```python
from build123d import *

# Parameters (mm, degrees)
SKETCH1_W                   = 14
SKETCH1_H                   = 16.3
SKETCH1_W_2                 = 10
SKETCH1_H_2                 = 13.3
SKETCH1_W_3                 = 9.5
SKETCH1_H_3                 = 7
CAP_EXTRUDE_DEPTH           = 1
SKETCH1_7_W                 = 14
SKETCH1_7_H                 = 5
FLAP_EXTRUDE_DEPTH          = 1.75
CUT_EXTRUDE2_REACH          = 3.75
SKETCH1_9_W                 = 9.5
SKETCH1_9_H                 = 7
F_1_5MM_DOWEL_HOLE1_D       = 1.5
F_1_5MM_DOWEL_HOLE1_DEPTH   = 1
TAP_DRILL_FOR_M2_TAP1_D     = 1.6
TAP_DRILL_FOR_M2_TAP1_DEPTH = 1.75


with BuildPart() as part:
    # Sketch1 → cap_extrude (new body)
    with BuildSketch(Plane.XY):
        Rectangle(SKETCH1_W, SKETCH1_H)
        Rectangle(SKETCH1_W_2, SKETCH1_H_2, mode=Mode.SUBTRACT)
        Rectangle(SKETCH1_W_2, SKETCH1_H_2)
        Rectangle(SKETCH1_W_3, SKETCH1_H_3, mode=Mode.SUBTRACT)
        Rectangle(SKETCH1_W_3, SKETCH1_H_3)
    extrude(amount=CAP_EXTRUDE_DEPTH)

    # Sketch1<7> → flap_extrude (add)
    with BuildSketch(Plane.XY):
        with Locations((0, 10.65)):
            Rectangle(SKETCH1_7_W, SKETCH1_7_H)
    extrude(amount=FLAP_EXTRUDE_DEPTH)

    # Sketch1<9> → Cut-Extrude2 (cut, up to next)
    with BuildSketch(Plane.XY, mode=Mode.PRIVATE) as cut_extrude2_sk1:
        Rectangle(SKETCH1_9_W, SKETCH1_9_H)
    cut_extrude2_tool1 = extrude(cut_extrude2_sk1.sketch, amount=CUT_EXTRUDE2_REACH, mode=Mode.PRIVATE) & part.part
    add(cut_extrude2_tool1.solids().sort_by_distance((0, 0, 0))[0], mode=Mode.SUBTRACT)

    # Ø1.5mm Dowel Hole1
    with Locations(Plane(origin=(0, 0, 0), x_dir=(-1, 0, 0), z_dir=(0, 0, -1))):
        with Locations((3.81, 6.65), (1.27, 6.65), (-1.27, 6.65), (-3.81, 6.65), (-3.81, -6.65), (-1.27, -6.65), (1.27, -6.65), (3.81, -6.65)):
            Hole(F_1_5MM_DOWEL_HOLE1_D / 2, depth=F_1_5MM_DOWEL_HOLE1_DEPTH)

    # Tap Drill for M2 Tap1
    with Locations(Plane(origin=(0, 0, 0), x_dir=(-1, 0, 0), z_dir=(0, 0, -1))):
        with Locations((-5, 11.15), (5, 11.15)):
            Hole(TAP_DRILL_FOR_M2_TAP1_D / 2, depth=TAP_DRILL_FOR_M2_TAP1_DEPTH)


solid = part.part
```
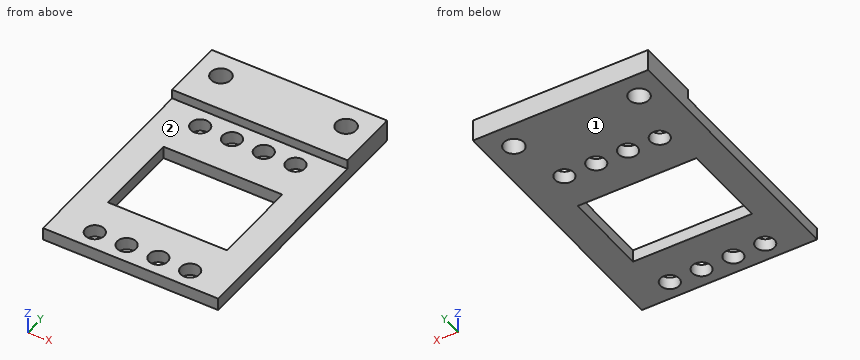
For this review, take the finished solid that the model builds, in its own axes (mm). Face numbers are marked on the shaded views. A direction names the side the tool comes from. Round coordinates to 2 decimals unless told otherwise and drop trailing zeros. Loops run counter-clockwise (first coordinate to the right, second up) from the corner with the lowest first, then second, coordinate; pieces in that order, holes last.
(1) Wall thickness on line 1 along Y through (x, z) = (-1.27, 0.65); line 2 along Y through (x, z) = (-3.5, 0.7); line 3 along Y through (x, z) = (-5, 1.5): over which ranges is each line inside the solid? List them lowest first.
Returned:
line 1: y = -8.15 to -7.4, -5.9 to -3.5, 3.5 to 5.9, 7.4 to 13.15
line 2: y = -8.15 to -7.33, -5.97 to -3.5, 3.5 to 5.97, 7.33 to 13.15
line 3: y = 8.15 to 10.35, 11.95 to 13.15
(2) Clearance check with flat-ended pins moving along their axes: P1, Ø0.9, axis at x = 1.27, y = -6.65, coming from the +Z side; P2, Ø8, axis at x = 2, y = -1, coming from the +Z side. State where each tip first meets the part, or that it passes through.
Returned:
P1: passes through
P2: stops at z = 1
(3) We need section D-D (y = 6.65). Give the boundary of the cut face in (x, z), plus the area to 3 significant figures.
Returned:
outline: (-7, 0) - (-4.56, 0) - (-4.56, 1) - (-7, 1) - close; (-3.06, 0) - (-2.02, 0) - (-2.02, 1) - (-3.06, 1) - close; (-0.52, 0) - (0.52, 0) - (0.52, 1) - (-0.52, 1) - close; (2.02, 0) - (3.06, 0) - (3.06, 1) - (2.02, 1) - close; (4.56, 0) - (7, 0) - (7, 1) - (4.56, 1) - close
area: 8.00 mm2
(4) Tool access review of the marked faces 1 and 2: name each direction out of +Z, -Z, +X, -X, +Y, -Y from which nothing blocks a thin tool from reaching the whole face with its end or side.
Returned:
face 1: -Z, +X, -X, +Y, -Y
face 2: +Z, +X, -X, -Y
(5) We need section B-B (z = 0.6). State how many separate pieces and enclosed holes the cut face has, plus the area to 3 significant figures.
Returned:
separate pieces: 1
enclosed holes: 11
area: 214 mm2
(6) We need section A-A (x = 0.25). Give the boundary of the cut face in (y, z).
Returned:
outline: (-8.15, 0) - (-3.5, 0) - (-3.5, 1) - (-8.15, 1) - close; (3.5, 0) - (13.15, 0) - (13.15, 1.75) - (8.15, 1.75) - (8.15, 1) - (3.5, 1) - close
(7) We need section C-C (y = -0.5). Give the boundary of the cut face in (x, z).
Returned:
outline: (-7, 0) - (-4.75, 0) - (-4.75, 1) - (-7, 1) - close; (4.75, 0) - (7, 0) - (7, 1) - (4.75, 1) - close
